The model under review builds one solid part; all positions refer to its coordinate system, in mm. A direction names the side the tool comes from. Coordinates: 2 decimals unless noted, no trailing zeros. Write each loop counter-clockwise with the first axis right and the second up, starting at its lowest first coordinate (ties: lowest second). Pieces come first, ordered by that corner, then holes. Notation, with made-up numbers: (-4, 3) -> (7, 3) arc R35 ccw to (7, 39) -> close; hole circle Ø7 at (-10, 31). An arc over 180 degrees is marked (long way). Put each result on its own line as item: value. Start each with the question number.
from build123d import *

# Parameters (mm, degrees)
SKETCH_1_R          = 2.575
EXTRUDE_1_DEPTH     = 55
SKETCH_2_W          = 35
SKETCH_2_H          = 35
EXTRUDE_2_DEPTH     = 2
SKETCH_8_R          = 1.15
CUT_EXTRUDE_5_DEPTH = 5
SKETCH_10_OUTSIDE_W = 51.798
SKETCH_10_OUTSIDE_H = 51.798
CUT_EXTRUDE_6_DEPTH = 5
SKETCH_14_R         = 1.15
CUT_EXTRUDE_7_DEPTH = 20


with BuildPart() as part:
    # 스케치1 → 보스-돌출1 (new body)
    with BuildSketch(Plane.XY):
        Circle(SKETCH_1_R)
    extrude(amount=EXTRUDE_1_DEPTH)

    # 스케치2 → 보스-돌출2 (add)
    with BuildSketch(Plane(origin=(0, 0, 0), x_dir=(-1, 0, 0), z_dir=(0, 0, -1))):
        Rectangle(SKETCH_2_W, SKETCH_2_H)
    extrude(amount=-EXTRUDE_2_DEPTH)

    # 스케치8 → 컷-돌출5 (cut)
    with BuildSketch(Plane(origin=(0, 0, 0), x_dir=(-1, 0, 0), z_dir=(0, 0, -1))):
        with Locations((13.533711803, 0)):
            Circle(SKETCH_8_R)
        with Locations((0, -13.533711803)):
            Circle(SKETCH_8_R)
        with Locations((-13.533711803, 0)):
            Circle(SKETCH_8_R)
        with Locations((0, 13.533711803)):
            Circle(SKETCH_8_R)
    extrude(amount=-CUT_EXTRUDE_5_DEPTH, mode=Mode.SUBTRACT)

    # 스케치10 outside → 컷-돌출6 (cut)
    with BuildSketch(Plane.XY.offset(2)):
        Rectangle(SKETCH_10_OUTSIDE_W, SKETCH_10_OUTSIDE_H)
        Polygon((-17.5, 0), (0, 17.5), (17.5, 0), (0, -17.5), align=None, mode=Mode.SUBTRACT)
    extrude(amount=-CUT_EXTRUDE_6_DEPTH, mode=Mode.SUBTRACT)

    # 스케치14 → 컷-돌출7 (cut)
    with BuildSketch(Plane(origin=(8.75, 8.75, 0), x_dir=(0.7071067811865475, -0.7071067811865477, 0), z_dir=(0.7071067811865477, 0.7071067811865475, 0))):
        with Locations(Location((0, -24.85, 0), (0, 0, 180))):
            Circle(SKETCH_14_R)
    extrude(amount=-CUT_EXTRUDE_7_DEPTH, mode=Mode.SUBTRACT)


solid = part.part
1. Tool access review of faces 4 (the cylindrical face through (2.456, 0.773, 28.129)), 5 (the cylindrical face through (14.683, 0.051, 0.986)): name each direction out of +Z, -Z, +X, -X, +Y, -Y from which nothing blocks a thin tool from reaching the whole face with its end or side.
2. Wall thickness on line 1 (Z direction, x = 8.5, y = 6.5); line 2 (Y direction, x = 0, z = 10) (3 decimals); line 3 (Y direction, x = 1, z = 45.5): over which ranges is each line inside the solid? List them lowest first. Write a range as from..to.
3. Consider section C-C on z = 27. State the section outline as (x, y) points (3 decimals), then the cut area to 3 significant figures.
4. Consider section A-A on y = -6. State the section outline as (x, z) points, then the cut area to 3 significant figures.
5. The part is to be moulded in two halves that separate along Z. For faces 1 (the cylindrical face through (-0.75, 0.8, 25.2)), 2 (the flat face through (8.9, -8.6, 1)), 3 (the flat face through (0, 0, 55)), say which applies: released by +Z, released by -Z, zero draft, split by the parting line, or undercut.
6. Consider section B-B on x = 10.5. State the section outline as (y, z) points.
7. Insertion check: P1, Ø4, axis at y = 3, z = 40, coming from the -X side; P2, Ø8, axis at x = 11.5, y = -7, coming from the +Z side; P3, Ø5, axis at x = -1.5, y = -7.5, coming from the -Z side; P4, Ø2, axis at x = 1.5, z = 26.5, coming from the -Y side. Each pin has a flat end and moves straight along its axis. Give the tip position at first contact, or say it passes through.
Output values:
1. face 4: +Z
1. face 5: +Z, -Z
2. line 1: z = 0..2
2. line 2: y = -2.575..2.575
2. line 3: y = -2.37..2.37
3. outline: circle Ø5.15 at (0, 0)
3. area: 20.8 mm^2
4. outline: (-11.5, 0) -> (11.5, 0) -> (11.5, 2) -> (-11.5, 2) -> close
4. area: 46.0 mm^2
5. face 1: undercut
5. face 2: zero draft
5. face 3: released by +Z
6. outline: (-7, 0) -> (7, 0) -> (7, 2) -> (-7, 2) -> close
7. P1: stops at x = -2.37
7. P2: stops at z = 2
7. P3: stops at z = 0
7. P4: stops at y = -2.53
